Part model, mm, in its own coordinate system. A direction names the side the tool comes from. Give positions to 0.01 mm unless a question says otherwise; leave off trailing zeros. Write each loop counter-clockwise with the first axis right and the second up, starting at its lowest first coordinate (ties: lowest second). Pieces come first, ordered by that corner, then holes. Notation, with made-up numbers: (12, -10.5) - (21, -10.5) arc R22 ccw to (21, 13.5) - close; hole circle Ø4 at (72.25, -10). An arc over 180 degrees is marked (long way). Answer as a JSON object with one key per item and string values. Group by question number.
Autodesk Inventor part; units mm, degrees
ref_plane "RWG-X" through (1.8795, 9, 10.525) normal (0, 0, -1) x (-1, 0, 0)
ref_plane "RWG-Y" through (0, 9, 9.585) normal (1, 0, 0) x (0, 0, -1)
ref_plane "YZ Plane" through (0, 0, 0) normal (1, 0, 0) x (0, 1, 0)
sketch "S-Basis" plane through (0, 0, 0) normal (0, 0, 1) x (1, 0, 0)
  line L0 (0, 57.19) -> (0, -57.19) construction
  line L1 (-56, 0) -> (56, 0) construction
  line L2 (-40, 40.85) -> (40, 40.85)
  line L3 (40, 40.85) -> (40, -40.85)
  line L4 (40, -40.85) -> (-40, -40.85)
  line L5 (-40, -40.85) -> (-40, 40.85)
  line L6 (-40, 40.85) -> (40, -40.85) construction
  line L7 (40, 40.85) -> (-40, -40.85) construction
  line L8 (-40, 33.35) -> (40, 33.35) construction
  circle A0 centre (-32.5, 33.35) radius 2.15
  circle A1 centre (32.5, 33.35) radius 2.15
  circle A2 centre (-32.5, -33.35) radius 2.15
  circle A3 centre (32.5, -33.35) radius 2.15
  line L9 (-4.418, 40.85) -> (4.418, 40.85)
  line L10 (-40, -40.85) -> (-16.2, -40.85) construction
  line L11 (-16.2, -40.85) -> (-16.2, -25.85) construction
  line L12 (-16.2, -25.85) -> (-40, -25.85) construction
  line L13 (-40, -25.85) -> (-40, -40.85) construction
  line L14 (-40, 40.85) -> (-16.2, 40.85) construction
  line L15 (-16.2, 40.85) -> (-16.2, 25.85) construction
  line L16 (-16.2, 25.85) -> (-40, 25.85) construction
  line L17 (-40, 25.85) -> (-40, 40.85) construction
  line L18 (40, -40.85) -> (16.2, -40.85) construction
  line L19 (16.2, -40.85) -> (16.2, -25.85) construction
  line L20 (16.2, -25.85) -> (40, -25.85) construction
  line L21 (40, -25.85) -> (40, -40.85) construction
  line L22 (40, 40.85) -> (16.2, 40.85) construction
  line L23 (40, 25.85) -> (40, 40.85) construction
  line L24 (16.2, 25.85) -> (40, 25.85) construction
  line L25 (16.2, 40.85) -> (16.2, 25.85) construction
  line L26 (-16.2, -35.85) -> (-14.2, -35.85)
  line L27 (-14.2, -35.85) -> (-14.2, -30.85)
  line L28 (-14.2, -30.85) -> (-16.2, -30.85)
  line L29 (-16.2, -30.85) -> (-16.2, -35.85)
  line L30 (-35, -25.85) -> (-30, -25.85)
  line L31 (-30, -25.85) -> (-30, -23.85)
  line L32 (-30, -23.85) -> (-35, -23.85)
  line L33 (-35, -23.85) -> (-35, -25.85)
  line L34 (-16.2, 35.85) -> (-14.2, 35.85)
  line L35 (-14.2, 35.85) -> (-14.2, 30.85)
  line L36 (-14.2, 30.85) -> (-16.2, 30.85)
  line L37 (-16.2, 30.85) -> (-16.2, 35.85)
  line L38 (-35, 25.85) -> (-30, 25.85)
  line L39 (-30, 25.85) -> (-30, 23.85)
  line L40 (-30, 23.85) -> (-35, 23.85)
  line L41 (-35, 23.85) -> (-35, 25.85)
  line L42 (16.2, -35.85) -> (14.2, -35.85)
  line L43 (14.2, -35.85) -> (14.2, -30.85)
  line L44 (14.2, -30.85) -> (16.2, -30.85)
  line L45 (16.2, -30.85) -> (16.2, -35.85)
  line L46 (35, -25.85) -> (30, -25.85)
  line L47 (30, -25.85) -> (30, -23.85)
  line L48 (30, -23.85) -> (35, -23.85)
  line L49 (35, -23.85) -> (35, -25.85)
  line L50 (14.2, 30.85) -> (16.2, 30.85)
  line L51 (14.2, 35.85) -> (14.2, 30.85)
  line L52 (16.2, 35.85) -> (14.2, 35.85)
  line L53 (16.2, 30.85) -> (16.2, 35.85)
  line L54 (30, 25.85) -> (30, 23.85)
  line L55 (30, 23.85) -> (35, 23.85)
  line L56 (35, 23.85) -> (35, 25.85)
  line L57 (35, 25.85) -> (30, 25.85)
  circle A4 centre (0, 0) radius 5.5
  circle A5 centre (0, 0) radius 6.3
  line L58 (0.6, 6.2714) -> (-0.6, 6.2714)
  line L59 (-0.6, 6.2714) -> (-0.6, 16.2714)
  line L60 (-0.6, 16.2714) -> (0.6, 16.2714)
  line L61 (0.6, 16.2714) -> (0.6, 6.2714)
  line L62 (-16.2714, -0.6) -> (-16.2714, 0.6)
  line L63 (-16.2714, 0.6) -> (-6.2714, 0.6)
  line L64 (-6.2714, -0.6) -> (-16.2714, -0.6)
  line L65 (-6.2714, 0.6) -> (-6.2714, -0.6)
  line L66 (0.6, -16.2714) -> (-0.6, -16.2714)
  line L67 (-0.6, -16.2714) -> (-0.6, -6.2714)
  line L68 (0.6, -6.2714) -> (0.6, -16.2714)
  line L69 (-0.6, -6.2714) -> (0.6, -6.2714)
  line L70 (16.2714, 0.6) -> (16.2714, -0.6)
  line L71 (16.2714, -0.6) -> (6.2714, -0.6)
  line L72 (6.2714, 0.6) -> (16.2714, 0.6)
  line L73 (6.2714, -0.6) -> (6.2714, 0.6)
  point P0 (0, 40.85)
  point P1 (-16.2, -33.35)
  point P2 (-16.2, 33.35)
  point P3 (16.2, -33.35)
  point P4 (16.2, 33.35)
  point P5 (-6.2714, -0.6)
  point P6 (-6.2714, -0.6)
  point P7 (-6.2714, 0.6)
  point P8 (-6.2714, 0.6)
  point P9 (6.2714, 0.6)
  point P10 (-0.6, -6.2714)
  point P11 (0.6, -6.2714)
  point P12 (6.2714, -0.6)
  dimension "d0" = 81.7
  dimension "d1" = 80
  dimension "d4" = 7.5
  dimension "d7" = 4.3
  dimension "d8" = 32.5
  dimension "d9" = 4.3
  dimension "d10" = 32.5
  dimension "d11" = 7.5
  dimension "d26" = 15
  dimension "d27" = 23.8
  dimension "d30" = 5
  dimension "d31" = 5
  dimension "d32" = 5
  dimension "d33" = 2
  dimension "d34" = 2
  dimension "d85" = 11
  dimension "d86" = 0.8
  dimension "d87" = 1.2
  dimension "d88" = 10
  dimension "d91" = 360
extrude "Ex-Base1" add sketch "S-Basis" against normal blind 2 contours L2 L3 L4 L5 | L29 L28 L27 L26 | L33 L32 L31 L30 | L34 L35 L36 L37 | L38 L39 L40 L41 | L42 L43 L44 L45 | L46 L47 L48 L49 | L51 L52 L53 L50 | L57 L56 L55 L54 | A5 L73 | A5 L72 L70 L71 | L73 A5 L69 L65 L58 | L58 A5 | A5 L59 L60 L61 | L68 L66 L67 A5 | A5 L69 | L65 A5 | A5 L64 L62 L63
extrude "Ex-Probe" [suppressed]
fillet "Rundung1" radius 2 4 edges at (40, -40.85, -1) (-40, -40.85, -1) (40, 40.85, -1) (-40, 40.85, -1)
ref_plane "RWG-X" through (1.8795, 9, 10.525) normal (0, 0, -1) x (-1, 0, 0)
ref_plane "RWG-Y" through (0, 9, 9.585) normal (1, 0, 0) x (0, 0, -1)
sketch "Skizze5" plane through (0, 0, 0) normal (0, 0, 1) x (1, 0, 0)
  line L0 (0, 57.19) -> (0, -57.19) construction
  line L1 (-35, -4) -> (-35, -20.85)
  line L2 (-35, -20.85) -> (-16.8473, -20.85)
  line L3 (-16.8473, -20.85) -> (-8, -4)
  line L4 (-8, -4) -> (-35, -4)
  line L5 (-11.2, -20.85) -> (-11.2, -35.85)
  line L6 (-11.2, -35.85) -> (-4, -35.85)
  line L7 (-4, -35.85) -> (-4, -7.1374)
  line L8 (-4, -7.1374) -> (-11.2, -20.85)
  line L9 (-56, 0) -> (56, 0) construction
  line L10 (35, -4) -> (35, -20.85)
  line L11 (35, -20.85) -> (16.8473, -20.85)
  line L12 (16.8473, -20.85) -> (8, -4)
  line L13 (8, -4) -> (35, -4)
  line L14 (11.2, -20.85) -> (11.2, -35.85)
  line L15 (11.2, -35.85) -> (4, -35.85)
  line L16 (4, -35.85) -> (4, -7.1374)
  line L17 (4, -7.1374) -> (11.2, -20.85)
  point P0 (0, 0)
  dimension "d74" = 4
  dimension "d77" = 5
  dimension "d78" = 4
extrude "Ex-ResinSave" cut sketch "Skizze5" against normal blind 2
fillet "Run-ResinSave" radius 2 4 edges at (-4, -7.1374, -1) (-8, -4, -1) (4, -7.1374, -1) (8, -4, -1)
mirror "Spiegeln3" about plane through (0, 0, 0) normal (0, 1, 0) of "Ex-ResinSave", "Run-ResinSave"
extrude "Ex-Führung" add sketch "S-Basis" along normal blind 40 contours A5 L73 | L73 A5 L69 L65 L58 | A5 L69
extrude "Ex-Stütze1" add sketch "S-Basis" along normal blind 40 contours L58 A5 | A5 L59 L60 L61
chamfer "Fase-Stütze1" distance 10 distance2 40 1 edges at (0, 16.2714, 40) measured on face at (0.2, 9.6047, 40)
pattern_circular "Runde Anordnung1" count 4 over 360 about axis through (0, 0, 0) along (0, 0, -1) of "Ex-Stütze1", "Fase-Stütze1"
equation "\"d10\" = d8"
equation "\"d11\" = d4"
properties part number "StiftHalter_PlateV1"
1) Saw through at A-A (y = 23). List the corners of the cut face in (x, z), and give its area (3 significant figures).
2) Saw through at C-C (z = 20). List the corners of the cut face in (x, y).
3) Two-plate mould, pull along X, no slides. Class faces 1 (the flat face through (0.01, -11.34, 19.72)), 2 (the cylindrical face through (-5.485, 13.316, -1.014)), 3 (the flat face through (-0.6, 10, 15)): +X half, -X half, draft (parallel to the pull), parting line (faces both ways), or undercut.
4) Which spindle directions (+Z, -Z, +X, -X, +Y, -Y) get a long thin tool onto all of the face, cutting with end or side? Do faces 4 (the flat face through (-1, 40.85, -1)), 5 (the cylindrical face through (-4.41, -4.5, 19.72)), 6 (the cylindrical face through (-4.5, 4.41, 19.72)), 7 (the flat face through (-0.01, 11.34, 19.72)), 8 (the flat face through (9.46, -17.54, -0.99)). Say none if no direction does.
5) Saw through at B-B (x = -27.5). List the corners of the cut face in (y, z).
6) Saw through at D-D (y = -33.35). List the corners of the cut face in (x, z).
7) Drop flat-ended pins along their axis: P1, Ø11, axis at x = 9, z = 24, coming from the +Y side; P2, Ø1.5, axis at x = -19.5, y = -24.5, coming from the +Z side; P3, Ø3, axis at x = -10.5, z = 11, coming from the -Y side. Give the stop position or say it passes through.
8) Drill centre lines: line 1 along Y through (x, z) = (-32.5, -1.5); line 2 along Y through (x, z) = (-32, -1); line 3 along Z through (x, y) = (2, -32). Where is each one in solid material? Low to high. Write a range as from..to.
Checks:
{
 "1": {"outline": "(-40, -2) - (-11.2, -2) - (-11.2, 0) - (-40, 0) - close; (-4, -2) - (4, -2) - (4, 0) - (-4, 0) - close; (11.2, -2) - (40, -2) - (40, 0) - (11.2, 0) - close", "area": "131 mm2"},
 "2": {"outline": "(-11.27, -0.6) - (-6.27, -0.6) arc R6.3 ccw to (-0.6, -6.27) - (-0.6, -11.27) - (0.6, -11.27) - (0.6, -6.27) arc R6.3 ccw to (6.27, -0.6) - (11.27, -0.6) - (11.27, 0.6) - (6.27, 0.6) arc R6.3 ccw to (0.6, 6.27) - (0.6, 11.27) - (-0.6, 11.27) - (-0.6, 6.27) arc R6.3 ccw to (-6.27, 0.6) - (-11.27, 0.6) - close; hole circle Ø11 at (0, 0)"},
 "3": {"face 1": "draft", "face 2": "undercut", "face 3": "-X half"},
 "4": {"face 4": "+Z, -Z, +X, -X, +Y", "face 5": "+Z, -X, -Y", "face 6": "+Z, -X, +Y", "face 7": "+Z, +X, -X, +Y", "face 8": "+Z, -Z"},
 "5": {"outline": "(-40.85, -2) - (-20.85, -2) - (-20.85, 0) - (-40.85, 0) - close; (-4, -2) - (4, -2) - (4, 0) - (-4, 0) - close; (20.85, -2) - (40.85, -2) - (40.85, 0) - (20.85, 0) - close"},
 "6": {"outline": "(-40, -2) - (-34.65, -2) - (-34.65, 0) - (-40, 0) - close; (-30.35, -2) - (-11.2, -2) - (-11.2, 0) - (-30.35, 0) - close; (-4, -2) - (4, -2) - (4, 0) - (-4, 0) - close; (11.2, -2) - (30.35, -2) - (30.35, 0) - (11.2, 0) - close; (34.65, -2) - (40, -2) - (40, 0) - (34.65, 0) - close"},
 "7": {"P1": "y = 5.24", "P2": "z = 0", "P3": "y = -0.6"},
 "8": {"line 1": "-40.85..-35.5, -31.2..-20.85, -4..4, 20.85..31.2, 35.5..40.85", "line 2": "-40.85..-35.44, -31.26..-20.85, -4..4, 20.85..31.26, 35.44..40.85", "line 3": "-2..0"}
}
